Design review of the part shown in the three views and the two pictorial views. Dimensions are in mm from the part's minimum x, y and z. Give positions to 0.01 mm unless a question says otherwise; leave off trailing zeros. Order: outer loops, then holes, each group sorted by start corner. A loop starts at its lowest first (then second) coordinate and runs counter-clockwise, first axis right, second up.
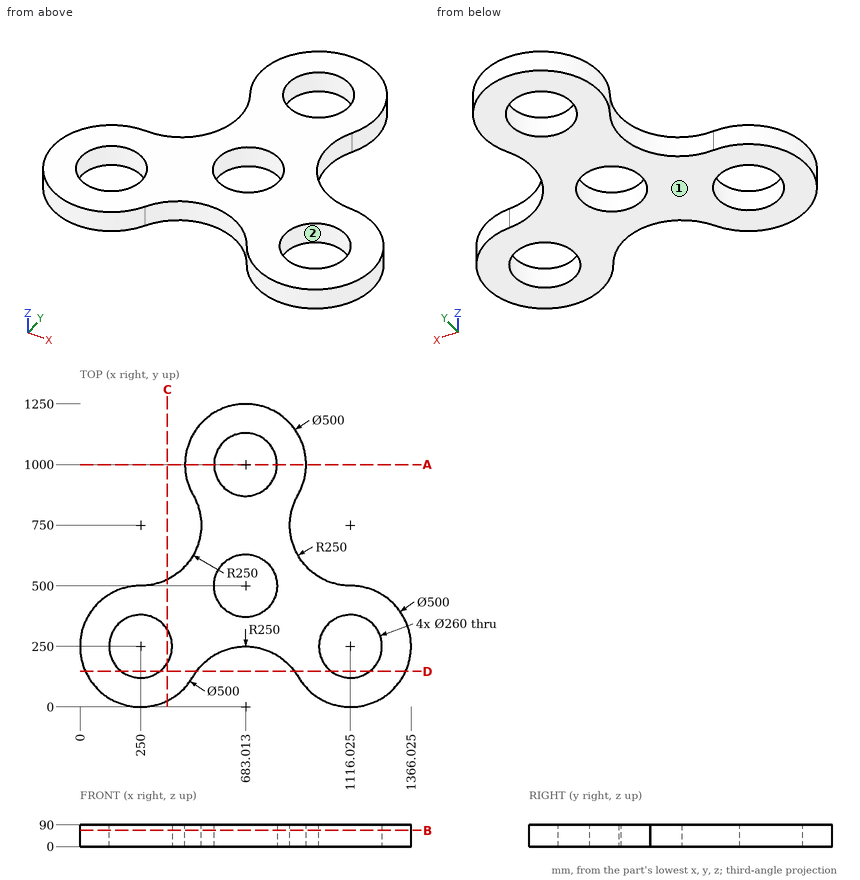
Item 1: For line 1 (Y direction, x = 625.5, z = 28.5) (1 decimal); line 2 (Y direction, x = 250, z = 22); line 3 (Y direction, x = 594.5, z = 52) (1 decimal), list the stretches that pass through material, from the lowest coordinate up.
Values found:
line 1: y = 243.3 to 383.4, 616.6 to 883.4, 1116.6 to 1243.3
line 2: y = 0 to 120, 380 to 500
line 3: y = 233.8 to 404.8, 595.2 to 904.8, 1095.2 to 1233.8
Item 2: Take a section at D-D (y = 146.5). Give the boundary of the cut face in (x, z) (1 decimal).
Values found:
outline: (22.4, 0) - (171.3, 0) - (171.3, 90) - (22.4, 90) - close; (328.7, 0) - (480.4, 0) - (480.4, 90) - (328.7, 90) - close; (885.6, 0) - (1037.4, 0) - (1037.4, 90) - (885.6, 90) - close; (1194.7, 0) - (1343.6, 0) - (1343.6, 90) - (1194.7, 90) - close
Item 3: Take a section at A-A (y = 1000). Give the boundary of the cut face in (x, z), and give its area (3 significant figures).
Values found:
outline: (433.01, 0) - (553.01, 0) - (553.01, 90) - (433.01, 90) - close; (813.01, 0) - (933.01, 0) - (933.01, 90) - (813.01, 90) - close
area: 21,600 mm2
Item 4: Take a section at B-B (z = 67.5). Give the boundary of the cut face in (x, y) (1 decimal).
Values found:
outline: (250, 500) arc R250 ccw (long way) to (466.5, 125) arc R250 cw to (899.5, 125) arc R250 ccw (long way) to (1116, 500) arc R250 cw to (899.5, 875) arc R250 ccw (long way) to (466.5, 875) arc R250 cw to start; hole circle Ø260 at (250, 250); hole circle Ø260 at (683, 500); hole circle Ø260 at (683, 1000); hole circle Ø260 at (1116, 250)
Item 5: Take a section at C-C (x = 361). Give the boundary of the cut face in (y, z), and give its area (3 significant figures).
Values found:
outline: (25.99, 0) - (182.33, 0) - (182.33, 90) - (25.99, 90) - close; (317.67, 0) - (525.99, 0) - (525.99, 90) - (317.67, 90) - close
area: 32,800 mm2
Item 6: Clearance check with flat-ended pins moving along their axes: pin 1 Ø3 at (x, z) = (1125.5, 22.5) entering from -Y; pin 2 Ø2 at (y, z) = (578.5, 21) entering from +X; pin 3 Ø1.5 at (y, z) = (186, 31.5) entering from +X; pin 4 Ø2 at (x, y) = (759, 353) entering from -Z. State where each tip first meets the part, or that it passes through.
Values found:
pin 1: stops at y = 0.13
pin 2: stops at x = 935.07
pin 3: stops at x = 1357.89
pin 4: stops at z = 0
Item 7: Draft analysis for pull direction X (two halves, no side actions). For the marked faces 1 and 2, state which applies: released by +X, released by -X, zero draft, split by the parting line, or undercut.
Values found:
face 1: zero draft
face 2: undercut
